For this review, take the finished solid that the model builds, in its own axes (mm). A direction names the side the tool comes from. Coordinates: 2 decimals unless noted, no trailing zeros. Order: outer loops, then holes, each group sorted by start corner. A loop starts at its lowest first (then second) coordinate and runs counter-clockwise, first axis right, second up.
Autodesk Inventor part; units mm, degrees
ref_plane "YZ Plane" through (0, 0, 0) normal (1, 0, 0) x (0, 1, 0)
ref_plane "XZ Plane" through (0, 0, 0) normal (0, 1, 0) x (-1, 0, 0)
ref_plane "XY Plane" through (0, 0, 0) normal (0, 0, 1) x (1, 0, 0)
sketch "Sketch1" plane through (0, 0, 0) normal (0, 0, 1) x (1, 0, 0)
  circle A0 centre (0, 0) radius 35
  dimension "d0" = 70
extrude "Extrusion1" add sketch "Sketch1" along normal blind 3
sketch "Sketch2" plane through (0, 0, 3) normal (0, 0, 1) x (1, 0, 0)
  circle A0 centre (0, 0) radius 2
  dimension "d3" = 4
extrude "Extrusion2" add sketch "Sketch2" along normal blind 24
sketch "Sketch3" plane through (0, 0, 27) normal (0, 0, 1) x (1, 0, 0)
  circle A0 centre (0, 0) radius 35
  dimension "d6" = 70
extrude "Extrusion3" add sketch "Sketch3" along normal blind 1
sketch "Sketch4" plane through (0, 0, 28) normal (0, 0, 1) x (1, 0, 0)
  circle A0 centre (0, 0) radius 1.1
  dimension "d9" = 2.2
extrude "Extrusion4" cut sketch "Sketch4" against normal through all
sketch "Sketch6" plane through (0, 0, 28) normal (0, 0, 1) x (1, 0, 0)
  circle A0 centre (0, 0) radius 2 construction
  circle A1 centre (-16.8114, -29.5) radius 0.4
  circle A2 centre (-2.5, 0) radius 0.4
  circle A3 centre (0, 0) radius 35
  dimension "d20" = 0.8
  dimension "d21" = 0.8
  dimension "d32" = 2.5
  dimension "d41" = 29.5
sketch "Sketch7" plane through (0, 0, 28) normal (0, 0, 1) x (1, 0, 0)
  point P0 (0, 0)
extrude "Extrusion5" cut sketch "Sketch6" against normal up to surface (1 mm away) contours A1 | A2
chamfer "Chamfer1" distance 0.4 angle 45 2 edges at (-2.9, 0, 28) (-17.2114, -29.5, 28)
sketch "Sketch9" plane through (0, 0, 0) normal (0, 0, -1) x (-1, 0, 0)
  point P0 (0, 0)
  point P1 (6.1, -7)
  point P2 (-24.1, -7)
  point P3 (-24.1, -12)
  point P4 (6.1, -12)
  dimension "d44" = 6.1
  dimension "d45" = 24.1
  dimension "d46" = 7
  dimension "d47" = 7
  dimension "d48" = 5
  dimension "d49" = 5
hole "Hole2" at (24.1, -7, 0) at (-6.1, -7, 0) at (24.1, -12, 0) at (-6.1, -12, 0) direction (0, 0, 1) diameter 2.459 depth 2.7
loft "Loft1" [suppressed]
properties part number "Bobbin_y_c"
1. Take a section at A-A, the plane x = 26.5. Give the boundary of the cut face in (y, z), plus the area to 3 significant figures.
Answer below:
outline: (-22.86, 0) - (22.86, 0) - (22.86, 3) - (-22.86, 3) - close; (-22.86, 27) - (22.86, 27) - (22.86, 28) - (-22.86, 28) - close
area: 183 mm2
2. To check wall thickness, follow L1, parallel to Z at x = -16, y = -22; L2, parallel to X at y = -12, z = 0.75; L3, parallel to Y at x = -6.1, z = 1.9. State the ranges of each line that lie inside material, in increasing order.
Answer below:
L1: z = 0 to 3, 27 to 28
L2: x = -32.88 to -7.33, -4.87 to 22.87, 25.33 to 32.88
L3: y = -34.46 to -13.23, -10.77 to -8.23, -5.77 to 34.46
3. Clearance check with flat-ended pins moving along their axes: pin 1 Ø1 at (x, z) = (19, 5) entering from -Y; pin 2 Ø2 at (x, y) = (24.1, -12) entering from -Z; pin 3 Ø6 at (x, z) = (3.5, 8.5) entering from +Y; pin 4 Ø2 at (y, z) = (2, 9.5) entering from +X. State where each tip first meets the part, or that it passes through.
Answer below:
pin 1: passes through
pin 2: stops at z = 2.7
pin 3: stops at y = 1.94
pin 4: stops at x = 1.73
4. Take a section at C-C, the plane z = 5. Give the boundary of the cut face in (x, y).
Answer below:
outline: circle Ø4 at (0, 0); hole circle Ø2.2 at (0, 0)
5. Take a section at B-B, the plane y = 6. Give the boundary of the cut face in (x, z), plus the area to 3 significant figures.
Answer below:
outline: (-34.48, 0) - (34.48, 0) - (34.48, 3) - (-34.48, 3) - close; (-34.48, 27) - (34.48, 27) - (34.48, 28) - (-34.48, 28) - close
area: 276 mm2
6. The part is to be moulded in two halves that separate along X. For faces 4 (the face through (24, -12, 2.7)), 5 (the face through (-27.77, 21.3, 27.49)), 6 (the face through (0, -7, 3)), 7 (the face through (-6, -7, 2.7)), say which applies: +X half, -X half, draft (parallel to the pull), parting line (faces both ways), or undercut.
Answer below:
face 4: undercut
face 5: parting line
face 6: draft
face 7: undercut
7. Machinability: for faces 1 (the face through (0, 2, 15)), 2 (the face through (0, -7, 0)), 3 (the face through (24, -7, 2.7)), which of the approach directions +Z, -Z, +X, -X, +Y, -Y give a long, thin tool a straight path to every point of the face, cutting with its end or side? Answer none if there is none.
Answer below:
face 1: none
face 2: -Z, +X, -X, +Y, -Y
face 3: -Z
8. Take a section at D-D, the plane y = -7. Give the boundary of the cut face in (x, z).
Answer below:
outline: (-34.29, 0) - (-7.33, 0) - (-7.33, 2.7) - (-4.87, 2.7) - (-4.87, 0) - (22.87, 0) - (22.87, 2.7) - (25.33, 2.7) - (25.33, 0) - (34.29, 0) - (34.29, 3) - (-34.29, 3) - close; (-34.29, 27) - (34.29, 27) - (34.29, 28) - (-34.29, 28) - close
